from build123d import *

# Parameters (mm, degrees)
BOSS_EXTRUDE1_DEPTH = 2
BOSS_EXTRUDE2_DEPTH = 7
SKETCH7_R           = 3
SKETCH7_R_2         = 1.100094
SKETCH7_R_3         = 1.100095
SKETCH7_R_4         = 1.14540164
SKETCH7_R_5         = 1.100094267
BOSS_EXTRUDE3_DEPTH = 4
CUT_EXTRUDE1_DEPTH  = 3
FILLET2_R           = 1
CHAMFER1_SIZE       = 0.5
CHAMFER2_SIZE       = 0.5


with BuildPart() as part:
    # Sketch3 → Boss-Extrude1 (new body)
    with BuildSketch(Plane.XY):
        with BuildLine():
            Line((60.855233133, 23.823211938), (47.949977192, 24.377676222))
            Line((47.949977192, 24.377676222), (9.438001399, 18.932389733))
            ThreePointArc((9.438001399, 18.932389733), (7.157815869, 19.520564151), (5.962231275, 21.549300871))
            Line((5.962231275, 21.549300871), (-1.970708405, 77.995680607))
            ThreePointArc((-1.970708405, 77.995680607), (-1.383464331, 80.271537635), (0.639738461, 81.467794829))
            Line((0.639738461, 81.467794829), (38.699898469, 86.902208152))
            Line((38.699898469, 86.902208152), (38.171393284, 94.460167157))
            ThreePointArc((38.171393284, 94.460167157), (38.910984807, 96.683773594), (41.002517903, 97.740613468))
            Line((41.002517903, 97.740613468), (60.921819416, 99.276682226))
            Line((60.921819416, 99.276682226), (60.921819416, 103.721902307))
            ThreePointArc((60.921819416, 103.721902307), (61.804499235, 105.878127499), (63.945786912, 106.796450874))
            Line((63.945786912, 106.796450874), (83.059551455, 107.113531682))
            ThreePointArc((83.059551455, 107.113531682), (85.251859467, 106.245869167), (86.185286941, 104.080744272))
            Line((86.185286941, 104.080744272), (86.24375422, 99.780452187))
            Line((86.24375422, 99.780452187), (154.596820419, 99.780452187))
            ThreePointArc((154.596820419, 99.780452187), (156.771169517, 98.879807301), (157.671814403, 96.705458202))
            Line((157.671814403, 96.705458202), (157.671814403, 14.057773112))
            ThreePointArc((157.671814403, 14.057773112), (157.497078938, 13.035997261), (156.992732263, 12.130352296))
            Line((156.992732263, 12.130352296), (146.547659954, -0.852593653))
            ThreePointArc((146.547659954, -0.852593653), (144.453525054, -1.98521487), (142.178510717, -1.283401812))
            Line((142.178510717, -1.283401812), (127.110775499, 11.324099062))
            Line((127.110775499, 11.324099062), (110.204782414, 17.079131321))
            Line((110.204782414, 17.079131321), (91.635796855, 16.870620568))
            Line((91.635796855, 16.870620568), (72.085555936, 14.46343429))
            ThreePointArc((72.085555936, 14.46343429), (70.725838171, 14.602041008), (69.560483965, 15.316179508))
            Line((69.560483965, 15.316179508), (60.855233133, 23.823211938))
        make_face()
    extrude(amount=BOSS_EXTRUDE1_DEPTH)

    # Sketch4 → Boss-Extrude2 (add)
    with BuildSketch(Plane.XY):
        with BuildLine():
            Line((47.949977192, 24.377676222), (60.855233133, 23.823211938))
            Line((60.855233133, 23.823211938), (69.560483965, 15.316179508))
            ThreePointArc((69.560483965, 15.316179508), (70.725838171, 14.602041008), (72.085555936, 14.46343429))
            Line((72.085555936, 14.46343429), (91.635796855, 16.870620568))
            Line((91.635796855, 16.870620568), (110.204782414, 17.079131321))
            Line((110.204782414, 17.079131321), (127.110775499, 11.324099062))
            Line((127.110775499, 11.324099062), (142.178510717, -1.283401812))
            ThreePointArc((142.178510717, -1.283401812), (144.453525054, -1.98521487), (146.547659954, -0.852593653))
            Line((146.547659954, -0.852593653), (156.992732263, 12.130352296))
            ThreePointArc((156.992732263, 12.130352296), (157.497078938, 13.035997261), (157.671814403, 14.057773112))
            Line((157.671814403, 14.057773112), (157.671814403, 96.705458202))
            ThreePointArc((157.671814403, 96.705458202), (156.771169517, 98.879807301), (154.596820419, 99.780452187))
            Line((154.596820419, 99.780452187), (86.24375422, 99.780452187))
            Line((86.24375422, 99.780452187), (86.185286941, 104.080744272))
            ThreePointArc((86.185286941, 104.080744272), (85.251859467, 106.245869167), (83.059551455, 107.113531682))
            Line((83.059551455, 107.113531682), (63.945786912, 106.796450874))
            ThreePointArc((63.945786912, 106.796450874), (61.804499235, 105.878127499), (60.921819416, 103.721902307))
            Line((60.921819416, 103.721902307), (60.921819416, 99.276682226))
            Line((60.921819416, 99.276682226), (41.002517903, 97.740613468))
            ThreePointArc((41.002517903, 97.740613468), (38.910984807, 96.683773594), (38.171393284, 94.460167157))
            Line((38.171393284, 94.460167157), (38.699898469, 86.902208152))
            Line((38.699898469, 86.902208152), (0.639738461, 81.467794829))
            ThreePointArc((0.639738461, 81.467794829), (-1.383464331, 80.271537635), (-1.970708405, 77.995680607))
            Line((-1.970708405, 77.995680607), (5.962231275, 21.549300871))
            ThreePointArc((5.962231275, 21.549300871), (7.157815869, 19.520564151), (9.438001399, 18.932389733))
            Line((9.438001399, 18.932389733), (47.949977192, 24.377676222))
        make_face()
        with BuildLine():
            ThreePointArc((84.258355662, 98.692914663), (84.533669024, 98.04695842), (85.183308419, 97.780452187))
            Line((85.183308419, 97.780452187), (154.596820419, 97.780452187))
            ThreePointArc((154.596820419, 97.780452187), (155.356955955, 97.465593738), (155.671814403, 96.705458202))
            Line((155.671814403, 96.705458202), (155.671814403, 14.057773112))
            ThreePointArc((155.671814403, 14.057773112), (155.610734868, 13.70060696), (155.434438315, 13.38403486))
            Line((155.434438315, 13.38403486), (144.989366006, 0.401088911))
            ThreePointArc((144.989366006, 0.401088911), (144.257272174, 0.005133041), (143.461944249, 0.250481615))
            Line((143.461944249, 0.250481615), (128.108249423, 13.097251096))
            Line((128.108249423, 13.097251096), (110.524936275, 19.082852408))
            Line((110.524936275, 19.082852408), (91.501949272, 18.869243682))
            Line((91.501949272, 18.869243682), (71.841145237, 16.448443965))
            ThreePointArc((71.841145237, 16.448443965), (71.365754809, 16.496904248), (70.958318613, 16.74658445))
            Line((70.958318613, 16.74658445), (61.958856362, 25.54112911))
            ThreePointArc((61.958856362, 25.54112911), (61.679828995, 25.728441638), (61.352295386, 25.803701118))
            Line((61.352295386, 25.803701118), (47.852081394, 26.383727313))
            Line((47.852081394, 26.383727313), (9.158002316, 20.91269287))
            ThreePointArc((9.158002316, 20.91269287), (8.360780393, 21.118336461), (7.942767807, 21.827644264))
            Line((7.942767807, 21.827644264), (0.009828128, 78.274024))
            ThreePointArc((0.009828128, 78.274024), (0.215128769, 79.069664055), (0.922440855, 79.487875801))
            Line((0.922440855, 79.487875801), (39.972806225, 85.063675424))
            ThreePointArc((39.972806225, 85.063675424), (40.561555536, 85.398058084), (40.76480024, 86.043913413))
            Line((40.76480024, 86.043913413), (40.166521363, 94.599680421))
            ThreePointArc((40.166521363, 94.599680421), (40.425084652, 95.377059525), (41.156290542, 95.746533736))
            Line((41.156290542, 95.746533736), (62.067941403, 97.359127107))
            ThreePointArc((62.067941403, 97.359127107), (62.675544492, 97.652931317), (62.921819416, 98.281303094))
            Line((62.921819416, 98.281303094), (62.921819416, 103.721902307))
            ThreePointArc((62.921819416, 103.721902307), (63.230393236, 104.475691655), (63.978960617, 104.796726017))
            Line((63.978960617, 104.796726017), (83.09272516, 105.113806824))
            ThreePointArc((83.09272516, 105.113806824), (83.859148665, 104.810474928), (84.185471769, 104.053554549))
            Line((84.185471769, 104.053554549), (84.258355662, 98.692914663))
        make_face(mode=Mode.SUBTRACT)
    extrude(amount=BOSS_EXTRUDE2_DEPTH)

    # Sketch7 → Boss-Extrude3 (add)
    # profile 1 of 6: a face of its own
    with BuildSketch(Plane.XY):
        with Locations((25.178343626, 43.435558637)):
            Circle(SKETCH7_R)
        with Locations((25.178343626, 43.435558637)):
            Circle(SKETCH7_R_2, mode=Mode.SUBTRACT)
    # profile 2 of 6: a face of its own
    with BuildSketch(Plane.XY):
        with Locations((22.534055897, 62.250653675)):
            Circle(SKETCH7_R)
        with Locations((22.534055897, 62.250653675)):
            Circle(SKETCH7_R_2, mode=Mode.SUBTRACT)
    # profile 3 of 6: a face of its own
    with BuildSketch(Plane.XY):
        with Locations((63.99681822, 84.705447078)):
            Circle(SKETCH7_R)
        with Locations((63.99681822, 84.705447078)):
            Circle(SKETCH7_R_3, mode=Mode.SUBTRACT)
    # profile 4 of 6: a face of its own
    with BuildSketch(Plane.XY):
        with Locations((73.496822591, 41.005447941)):
            Circle(SKETCH7_R)
        with Locations((73.496822591, 41.005447941)):
            Circle(SKETCH7_R_3, mode=Mode.SUBTRACT)
    # profile 5 of 6: a face of its own
    with BuildSketch(Plane.XY):
        with Locations((124.796820928, 64.405450202)):
            Circle(SKETCH7_R)
        with Locations((124.796820928, 64.405450202)):
            Circle(SKETCH7_R_4, mode=Mode.SUBTRACT)
    # profile 6 of 6: a face of its own
    with BuildSketch(Plane.XY):
        with Locations((134.70931431, 21.546419059)):
            Circle(SKETCH7_R)
        with Locations((134.70931431, 21.546419059)):
            Circle(SKETCH7_R_5, mode=Mode.SUBTRACT)
    extrude(amount=BOSS_EXTRUDE3_DEPTH)

    # Sketch8 → Cut-Extrude1 (cut)
    with BuildSketch(Plane(origin=(157.671814403, 0, 0), x_dir=(0, 0, -1), z_dir=(1, 0, 0))):
        with BuildLine():
            Line((-1, 62.669458202), (-1, 54.541458202))
            ThreePointArc((-1, 54.541458202), (-3.061576359, 52.479881843), (-5.123152718, 54.541458202))
            Line((-5.123152718, 54.541458202), (-5.123152718, 62.669458202))
            ThreePointArc((-5.123152718, 62.669458202), (-3.061576359, 64.731034561), (-1, 62.669458202))
        make_face()
    extrude(amount=-CUT_EXTRUDE1_DEPTH, mode=Mode.SUBTRACT)

    # Fillet2
    fillet2_edges = [part.edges().sort_by_distance(p)[0] for p in [
        (65.207858549, 19.569695723, 0),
        (54.402605163, 24.10044408, 0),
        (28.693989296, 21.655032978, 0),
        (7.157815869, 19.520564151, 0),
        (1.995761435, 49.772490739, 0),
        (-1.383464331, 80.271537635, 0),
        (19.669818465, 84.18500149, 0),
        (38.435645877, 90.681187654, 0),
        (38.910984807, 96.683773594, 0),
        (50.962168659, 98.508647847, 0),
        (60.921819416, 101.499292266, 0),
        (61.804499235, 105.878127499, 0),
        (73.502669184, 106.954991278, 0),
        (85.251859467, 106.245869167, 0),
        (86.21452058, 101.930598229, 0),
        (120.420287319, 99.780452187, 0),
        (156.771169517, 98.879807301, 0),
        (157.671814403, 55.381615657, 0),
        (157.497078938, 13.035997261, 0),
        (151.770196108, 5.638879321, 0),
        (144.453525054, -1.98521487, 0),
        (134.644643108, 5.020348625, 0),
        (118.657778957, 14.201615191, 0),
        (100.920289635, 16.974875944, 0),
        (81.860676395, 15.667027429, 0),
        (70.725838171, 14.602041008, 0),
    ]]
    fillet(fillet2_edges, radius=FILLET2_R - 0.0001)  # a hair under: the kernel refuses the full size

    # Chamfer1
    chamfer1_edges = [part.edges().sort_by_distance(p)[0] for p in [
        (70.725838171, 14.602041008, 7),
        (81.860676395, 15.667027429, 7),
        (100.920289635, 16.974875944, 7),
        (118.657778957, 14.201615191, 7),
        (134.644643108, 5.020348625, 7),
        (144.453525054, -1.98521487, 7),
        (151.770196108, 5.638879321, 7),
        (157.497078938, 13.035997261, 7),
        (157.671814403, 55.381615657, 7),
        (156.771169517, 98.879807301, 7),
        (120.420287319, 99.780452187, 7),
        (86.21452058, 101.930598229, 7),
        (85.251859467, 106.245869167, 7),
        (73.502669184, 106.954991278, 7),
        (61.804499235, 105.878127499, 7),
        (60.921819416, 101.499292266, 7),
        (50.962168659, 98.508647847, 7),
        (38.910984807, 96.683773594, 7),
        (38.435645877, 90.681187654, 7),
        (19.669818465, 84.18500149, 7),
        (-1.383464331, 80.271537635, 7),
        (1.995761435, 49.772490739, 7),
        (7.157815869, 19.520564151, 7),
        (28.693989296, 21.655032978, 7),
        (54.402605163, 24.10044408, 7),
        (65.207858549, 19.569695723, 7),
    ]]
    chamfer(chamfer1_edges, length=CHAMFER1_SIZE)

    # Chamfer2
    chamfer2_edges = [part.edges().sort_by_distance(p)[0] for p in [
        (133.609220043, 21.546419059, 4),
        (123.651419288, 64.405450202, 4),
        (72.396727591, 41.005447941, 4),
        (62.89672322, 84.705447078, 4),
        (21.433961897, 62.250653675, 4),
        (24.078249626, 43.435558637, 4),
    ]]
    chamfer(chamfer2_edges, length=CHAMFER2_SIZE)


solid = part.part
Geometry check sheet. Reference: the model listing, model coordinates, mm. A direction names the side the tool comes from. Give positions to 0.01 mm unless a question says otherwise; leave off trailing zeros. Write each question's results on one line, items separated by ' | '.
1) Gauge pin test, flat ends, axial feed: pin 1 (1.5 mm diameter, centred on x = 155.5, y = 57.5, fed in from +Z); pin 2 (2.5 mm diameter, centred on x = 124.5, y = 64.5, fed in from +Z); pin 3 (6.5 mm diameter, centred on x = 25, y = 44.5, fed in from +Z); pin 4 (3.5 mm diameter, centred on y = 102.5, z = 4, fed in from -X). Record the tip position at first contact, or that the pin passes through.
Answers follow:
pin 1: z = 7 | pin 2: z = 3.92 | pin 3: z = 4 | pin 4: x = 60.92
2) Thickness scan on line 1 (Z direction, x = 63, y = 76); line 2 (X direction, y = 77, z = 2.75); line 3 (X direction, y = 11, z = 2.5). Record the ranges inside material, lowest first.
Answers follow:
line 1: 0 to 2 | line 2: -1.83 to 0.19, 155.67 to 157.67 | line 3: 127.5 to 130.61, 153.52 to 156.08
3) Release check for a two-part mould opening along Y. For faces 5 (the face through (61.781, 105.854, 3.711)), 6 (the face through (134.666, 5.333, 6.753)), 7 (the face through (75, 40, 4)) record: +Y half, -Y half, draft (parallel to the pull), parting line (faces both ways), or undercut.
Answers follow:
face 5: +Y half | face 6: -Y half | face 7: undercut
4) Tool access check on faces 1 (the face through (50.823, 98.498, 3.711)), 2 (the face through (81.714, 15.952, 0.285)), 3 (the face through (65.3, 19.9, 6.8)), 4 (the face through (66.522, 21.082, 4.465)). Record the directions out of +Z, -Z, +X, -X, +Y, -Y that give a thin tool (end or side, any length) a straight path to the whole face; none if there is none.
Answers follow:
face 1: +Z, -Z, -X, +Y | face 2: -Z, -Y | face 3: +Z, -Y | face 4: +Z
